Geometry: see drawing. Coordinates: mm, zero at the bounding-box minimum. Give positions to 0.01 mm unless a question says otherwise; leave off trailing zeros. Write each loop counter-clockwise with the first axis right and the second up, starting at its lowest first coordinate (ties: lowest second). Pieces come first, ordered by that corner, then holes. Notation, with made-up numbers: (63, -14.5) - (98, -14.5) arc R21 ccw to (98, -0.5) - close; hole circle Ø9 at (-29.75, -15). An arc over 180 degrees is marked (long way). Return JSON: item names as keys, results as strings.
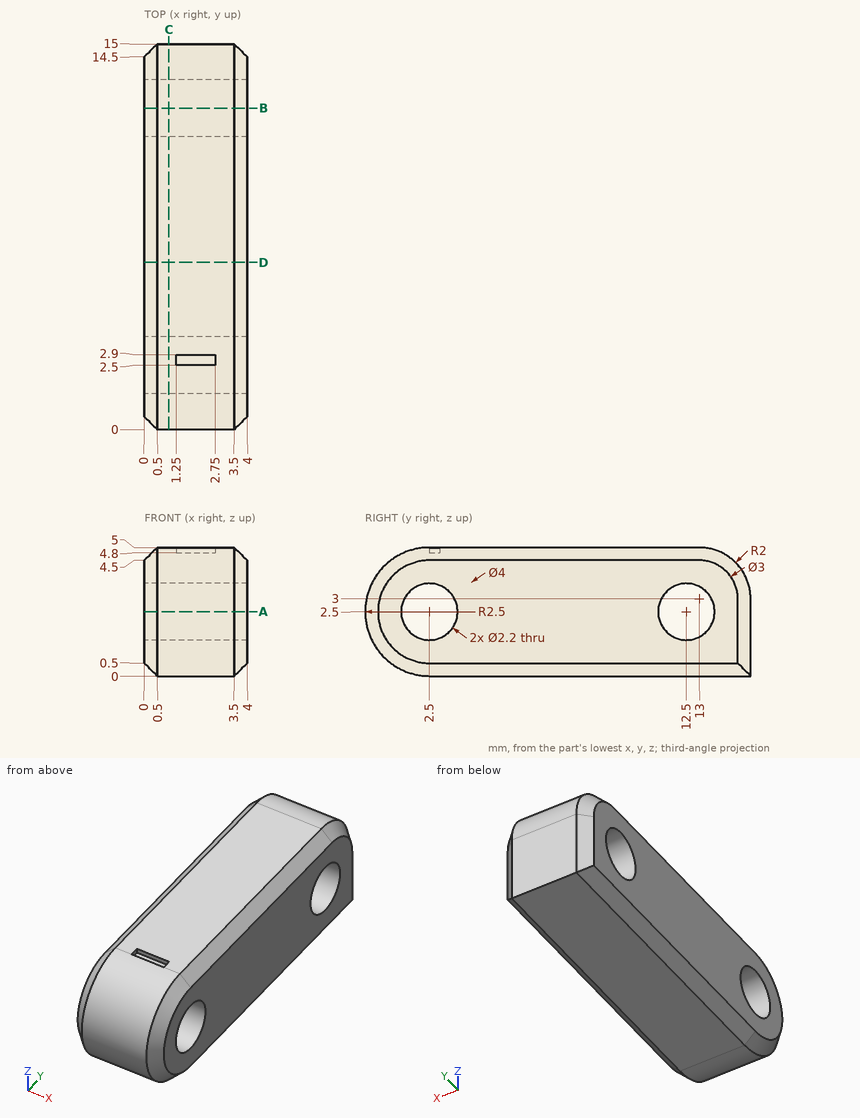
Q1. Section query D-D, the plane y = 6.5. Return the cut outline in (x, z), plus the area to 3 significant figures.
Answer key:
{"outline": "(0, 0.5) - (0.5, 0) - (3.5, 0) - (4, 0.5) - (4, 4.5) - (3.5, 5) - (0.5, 5) - (0, 4.5) - close", "area": "19.5 mm^2"}
Q2. Pin query (flat end, axial travel): P1, Ø2, axis at y = 12.5, z = 2.5, coming from the -X side; P2, Ø1.5, axis at x = 2, y = 13.5, coming from the -Z side. Return the tip coordinate at first contact, or that it passes through.
Answer key:
{"P1": "passes through", "P2": "stops at z = 0"}
Q3. Material intervals for probe 1 along Z at (x, y) = (0.8, 12.5); probe 2 along Y at (x, z) = (1.5, 2.85); probe 3 along Y at (x, z) = (0.7, 2.8), sorted ascending. Write a range as [from, to].
Answer key:
{"probe 1": "z = [0, 1.4], [3.6, 5]", "probe 2": "y = [0.02, 1.46], [3.54, 11.46], [13.54, 15]", "probe 3": "y = [0.02, 1.44], [3.56, 11.44], [13.56, 15]"}
Q4. Section query C-C, the plane x = 0.95. Return the cut outline in (y, z).
Answer key:
{"outline": "(2.5, 0) - (15, 0) - (15, 3) arc R2 ccw to (13, 5) - (2.5, 5) arc R2.5 ccw to start; hole circle Ø2.2 at (2.5, 2.5); hole circle Ø2.2 at (12.5, 2.5)"}
Q5. Section query A-A, the plane z = 2.5. Return the cut outline in (x, y), plus the area to 3 significant figures.
Answer key:
{"outline": "(0, 0.5) - (0.5, 0) - (3.5, 0) - (4, 0.5) - (4, 1.4) - (0, 1.4) - close; (0, 3.6) - (4, 3.6) - (4, 11.4) - (0, 11.4) - close; (0, 13.6) - (4, 13.6) - (4, 14.5) - (3.5, 15) - (0.5, 15) - (0, 14.5) - close", "area": "41.9 mm^2"}
Q6. Section query B-B, the plane y = 12.5. Return the cut outline in (x, z).
Answer key:
{"outline": "(0, 0.5) - (0.5, 0) - (3.5, 0) - (4, 0.5) - (4, 1.4) - (0, 1.4) - close; (0, 3.6) - (4, 3.6) - (4, 4.5) - (3.5, 5) - (0.5, 5) - (0, 4.5) - close"}
